For this review, take the finished solid that the model builds, in its own axes (mm). Round coordinates to 2 decimals unless told otherwise and drop trailing zeros. Write each loop counter-clockwise with the first axis right and the second up, starting at its lowest first coordinate (ties: lowest second). Pieces come first, ordered by that corner, then holes. Notation, with made-up numbers: (-29.5, -37) -> (9.5, -37) arc R17 ccw to (9.5, -7) -> close; hole circle Ø9 at (-33.5, 82.5). An arc over 180 degrees is marked (long way). Answer as CSV lines item,"result". Start each with the question number.
Item 1: Take a section at D-D on z = 2.25. Count the separate pieces of the cut face and the enclosed holes in it, then the cut area to 3 significant figures.
Item 2: For pin 1 Ø1 at (x, y) = (-44, 38.5) entering from -Z; pin 2 Ø4 at (x, y) = (-82, 93) entering from -Z, all flat-tipped, find the tip position at first contact; note any pin that passes through.
Item 3: Wall thickness on probe 1 along Y at (x, z) = (45, 1); probe 2 along Y at (x, z) = (-81, 0.8); probe 3 along X at (y, z) = (-46, 2.55): over which ranges is each line inside the solid? List them lowest first. Write a range as from..to.
Item 4: Take a section at C-C on y = 93. Give the boundary of the cut face in (x, z), then the cut area to 3 significant figures.
Item 5: Mouldability with a two-part tool opening along Y and no side actions: class faces 1 (the cylindrical face through (-84.1, 93.09, 1.48)), 2 (the flat face through (-20, 1, 0)) as +Y half, -Y half, draft (parallel to the pull), parting line (faces both ways), or undercut.
Item 6: Take a section at B-B on x = 45. Give the boundary of the cut face in (y, z).
Item 7: Take a section at A-A on y = -76. Give the boundary of the cut face in (x, z).
```python
from build123d import *

# Parameters (mm, degrees)
SERVICE_LID_VENTS_PROFILE_W = 145
SERVICE_LID_VENTS_PROFILE_H = 198
SERVICE_LID_VENTS_PROFILE_R = 2.1
SERVICE_LID_VENTS_DEPTH     = 3


with BuildPart() as part:
    # Service lid vents profile → Service lid vents (new body)
    with BuildSketch(Plane.XY):
        with Locations((-18.5, 0)):
            Rectangle(SERVICE_LID_VENTS_PROFILE_W, SERVICE_LID_VENTS_PROFILE_H)
        with Locations((-82, -93)):
            Circle(SERVICE_LID_VENTS_PROFILE_R, mode=Mode.SUBTRACT)
        with Locations((-82, 93)):
            Circle(SERVICE_LID_VENTS_PROFILE_R, mode=Mode.SUBTRACT)
        with Locations((45, -93)):
            Circle(SERVICE_LID_VENTS_PROFILE_R, mode=Mode.SUBTRACT)
        with Locations((45, 93)):
            Circle(SERVICE_LID_VENTS_PROFILE_R, mode=Mode.SUBTRACT)
        with BuildLine():
            Line((-33, -78.5), (21, -78.5))
            ThreePointArc((21, -78.5), (23.5, -76), (21, -73.5))
            Line((21, -73.5), (-33, -73.5))
            ThreePointArc((-33, -73.5), (-35.5, -76), (-33, -78.5))
        make_face(mode=Mode.SUBTRACT)
        with BuildLine():
            Line((-33, -63.5), (21, -63.5))
            ThreePointArc((21, -63.5), (23.5, -61), (21, -58.5))
            Line((21, -58.5), (-33, -58.5))
            ThreePointArc((-33, -58.5), (-35.5, -61), (-33, -63.5))
        make_face(mode=Mode.SUBTRACT)
        with BuildLine():
            Line((-33, -48.5), (21, -48.5))
            ThreePointArc((21, -48.5), (23.5, -46), (21, -43.5))
            Line((21, -43.5), (-33, -43.5))
            ThreePointArc((-33, -43.5), (-35.5, -46), (-33, -48.5))
        make_face(mode=Mode.SUBTRACT)
        with BuildLine():
            Line((-33, 43.5), (21, 43.5))
            ThreePointArc((21, 43.5), (23.5, 46), (21, 48.5))
            Line((21, 48.5), (-33, 48.5))
            ThreePointArc((-33, 48.5), (-35.5, 46), (-33, 43.5))
        make_face(mode=Mode.SUBTRACT)
        with BuildLine():
            Line((-33, 58.5), (21, 58.5))
            ThreePointArc((21, 58.5), (23.5, 61), (21, 63.5))
            Line((21, 63.5), (-33, 63.5))
            ThreePointArc((-33, 63.5), (-35.5, 61), (-33, 58.5))
        make_face(mode=Mode.SUBTRACT)
        with BuildLine():
            Line((-33, 73.5), (21, 73.5))
            ThreePointArc((21, 73.5), (23.5, 76), (21, 78.5))
            Line((21, 78.5), (-33, 78.5))
            ThreePointArc((-33, 78.5), (-35.5, 76), (-33, 73.5))
        make_face(mode=Mode.SUBTRACT)
    extrude(amount=SERVICE_LID_VENTS_DEPTH)


solid = part.part
```
Output values:
1,separate pieces,"1"
1,enclosed holes,"10"
1,area,"26,900 mm^2"
2,pin 1,"stops at z = 0"
2,pin 2,"passes through"
3,probe 1,"y = -99..-95.1, -90.9..90.9, 95.1..99"
3,probe 2,"y = -99..-94.85, -91.15..91.15, 94.85..99"
3,probe 3,"x = -91..-35.5, 23.5..54"
4,outline,"(-91, 0) -> (-84.1, 0) -> (-84.1, 3) -> (-91, 3) -> close; (-79.9, 0) -> (42.9, 0) -> (42.9, 3) -> (-79.9, 3) -> close; (47.1, 0) -> (54, 0) -> (54, 3) -> (47.1, 3) -> close"
4,area,"410 mm^2"
5,face 1,"undercut"
5,face 2,"draft"
6,outline,"(-99, 0) -> (-95.1, 0) -> (-95.1, 3) -> (-99, 3) -> close; (-90.9, 0) -> (90.9, 0) -> (90.9, 3) -> (-90.9, 3) -> close; (95.1, 0) -> (99, 0) -> (99, 3) -> (95.1, 3) -> close"
7,outline,"(-91, 0) -> (-35.5, 0) -> (-35.5, 3) -> (-91, 3) -> close; (23.5, 0) -> (54, 0) -> (54, 3) -> (23.5, 3) -> close"
